Can you work these out from the model? Positions are in its coordinate system, mm. A direction names the side the tool comes from. Coordinates: 2 decimals unless noted, no trailing zeros. Order: outer loops, then holes, each group sorted by start corner. A loop starts at its lowest first (then second) coordinate and runs counter-clockwise, first axis right, second up. Notation, with made-up numbers: M 79,55 L 114,55 A15 ccw 114,77 Z; hole C 20,80.25 d7. An arc over 180 degrees is marked long. Answer as a JSON object with one key per item and string values.
from build123d import *

# Parameters (mm, degrees)
F1_DEPTH = 10
F3_DEPTH = 1
F4_SIZE  = 1


with BuildPart() as f1:
    # F0 (on Front) → F1 (new body)
    with BuildSketch(Plane.XZ):
        Polygon((0, 20), (0, 50), (-25, 0), (-17.5, 0), (-7.5, 20), (-7.5, 5), align=None)
    extrude(amount=F1_DEPTH)

    # F2 (on face) → F3 (join)
    with BuildSketch(Plane(origin=(0, 0, 0), x_dir=(1, 0, 0), z_dir=(0, 0, -1))):
        Polygon((-21.25, 7.5), (-23.75, 7.5), (-23.75, 5), (-23.75, 2.5), (-21.25, 2.5), (-18.75, 2.5), (-18.75, 5), (-18.75, 7.5), align=None)
    extrude(amount=F3_DEPTH)

    # F4
    f4_edges = [f1.edges().sort_by_distance(p)[0] for p in [
        (-12.5, -10, 25),
        (0, -10, 35),
        (-12.5, 0, 25),
        (0, 0, 35),
        (-12.5, -10, 10),
        (-7.5, -10, 12.5),
        (-12.5, 0, 10),
        (-7.5, 0, 12.5),
        (-3.75, -10, 12.5),
        (-3.75, 0, 12.5),
    ]]
    chamfer(f4_edges, length=F4_SIZE)


solid = f1.part
Item 1: I want a section at A-A, the plane z = 11. Write out the boundary of the cut face in (x, y).
Answers follow:
{"outline": "M -19.5,-9 L -18.38,-10 L -13.12,-10 L -12,-9 L -12,-1 L -13.12,0 L -18.38,0 L -19.5,-1 Z; M -7.5,-9 L -6.5,-10 L -5.62,-10 L -4.5,-9 L -4.5,-1 L -5.62,0 L -6.5,0 L -7.5,-1 Z"}
Item 2: Please list where these lines run through material, in increasing order: line 1 (X direction, y = -3.75, z = 15); line 2 (X direction, y = -2.5, z = 8); line 3 (Z direction, x = -21.5, y = -1.75).
Answers follow:
{"line 1": "x = -17.5 to -10, -7.5 to -2.5", "line 2": "x = -21 to -13.5, -7.5 to -6", "line 3": "z = 0 to 7"}
Item 3: I'm going to push flat-ended pins straight in: pin 1 (5 mm diameter, centred on y = -7.5, z = 5, fed in from +X); pin 2 (1 mm diameter, centred on x = -12, y = -6.5, fed in from -Z); pin 3 (3 mm diameter, centred on x = -22.5, y = -2.5, fed in from +Z). Where does each tip first touch, or does it pass through?
Answers follow:
{"pin 1": "stops at x = -6.25", "pin 2": "stops at z = 10", "pin 3": "stops at z = 8"}
Item 4: If we mould it in two halves opening along X, with no side actions, what happens to faces 1 (the flat face through (-12.57, -4.94, 9.86)), 2 (the flat face through (-3.423, -9.507, 14.288)), 3 (the flat face through (-24, -5, 0))? For each: pulls with the +X half, pulls with the -X half, needs draft (parallel to the pull), parting line crosses it, or undercut.
Answers follow:
{"face 1": "undercut", "face 2": "pulls with the +X half", "face 3": "needs draft"}
Item 5: I want a section at D-D, the plane z = 25.5. Write out the boundary of the cut face in (x, y), plus the area to 3 significant figures.
Answers follow:
{"outline": "M -12.25,-9 L -11.13,-10 L -1,-10 L 0,-9 L 0,-1 L -1,0 L -11.13,0 L -12.25,-1 Z", "area": "120 mm^2"}
Item 6: I want a section at B-B, the plane y = -3.5. Write out the boundary of the cut face in (x, z), plus the area to 3 significant figures.
Answers follow:
{"outline": "M -25,0 L -23.75,0 L -23.75,-1 L -18.75,-1 L -18.75,0 L -17.5,0 L -7.5,20 L -7.5,5 L 0,20 L 0,50 Z", "area": "436 mm^2"}
Item 7: I want a section at C-C, the plane x = -22.25. Write out the boundary of the cut face in (y, z).
Answers follow:
{"outline": "M -10,0 L -7.5,0 L -7.5,-1 L -2.5,-1 L -2.5,0 L 0,0 L 0,3.26 L -1,5.5 L -9,5.5 L -10,3.26 Z"}
Item 8: Which directions (+Z, -Z, +X, -X, +Y, -Y) give clear straight access to the entire face, cutting with the end or side of a thin tool? Please do faces 4 (the flat face through (-21.2, -7.5, -0.5)), 5 (the flat face through (-7.5, -5, 13)), 6 (the flat face through (-23.75, -5, -0.5)).
Answers follow:
{"face 4": "-Z, +X, -X, -Y", "face 5": "-Z, +Y, -Y", "face 6": "-Z, -X, +Y, -Y"}
